Model file for the job. Use its own axes, mm. Coordinates: 2 decimals unless noted, no trailing zeros. Write each loop counter-clockwise with the first axis right and the second up, starting at its lowest first coordinate (ties: lowest second). Pieces come first, ordered by that corner, then holes.
Q1. Band-saw the part on A-A, the plane x = 25.4. Write the cut outline in (y, z) (1 decimal).
Q2. Band-saw the part on C-C, the plane y = -1.1. State how many separate pieces and enclosed holes the cut face has, plus the area to 3 significant figures.
Q3. Drill centre lines: probe 1 along X at (y, z) = (-2.25, -12.7); probe 2 along Z at (x, y) = (43.5, -2.65); probe 3 along X at (y, z) = (-2.1, -88) (3 decimals). Where is each one in solid material? Low to high.
Q4. Band-saw the part on B-B, the plane z = -12.7. Write the cut outline in (x, y) (3 decimals).
Q5. Band-saw the part on D-D, the plane x = 38.1. Write the cut outline in (y, z) (1 decimal), plus the area to 3 significant figures.
Q6. Pin check, flat tips, straight feed: P1, Ø1.6, axis at y = -1.5, z = -61, coming from the -X side (3 decimals); P2, Ø1, axis at x = 8, y = -1, coming from the -Z side; P3, Ø8, axis at x = 50.8, z = -87.31, coming from the +Y side; P4, Ø1.6, axis at y = -2, z = -85, coming from the -X side (3 decimals). Stop position of each tip, or through.
from build123d import *

# Parameters (mm, degrees)
SKETCH1_W          = 82.55
SKETCH1_H          = 96.8375
SKETCH1_W_2        = 38.1
SKETCH1_H_2        = 38.1
BASE_FLANGE2_DEPTH = 3.175
SKETCH3_W          = 12.7
SKETCH3_H          = 71.4375
CUT_EXTRUDE2_DEPTH = 128.287409162
SKETCH2_R          = 2.54
CUT_EXTRUDE1_DEPTH = 128.287409162
SKETCH5_W          = 15.875
SKETCH5_H          = 53.975
CUT_EXTRUDE6_DEPTH = 128.287409162
SKETCH7_R          = 2.54
CUT_EXTRUDE7_DEPTH = 128.287409162


# Sheet-metal steps are written as plain solids
with BuildPart() as part:
    # Base-Flange2: sheet metal written as solids
    # Sketch1 → Base-Flange2 (new body)
    with BuildSketch(Plane(origin=(0, 0, 0), x_dir=(1, 0, 0), z_dir=(0, 1, 0))):
        with Locations((41.275, 48.41875)):
            Rectangle(SKETCH1_W, SKETCH1_H)
        with Locations((47.625, 61.9125)):
            Rectangle(SKETCH1_W_2, SKETCH1_H_2, mode=Mode.SUBTRACT)
    extrude(amount=-BASE_FLANGE2_DEPTH)

    # Sketch3 → Cut-Extrude2 (cut, through all)
    with BuildSketch(Plane(origin=(0, 0, 0), x_dir=(1, 0, 0), z_dir=(0, 1, 0))):
        with Locations((6.35, 61.11875)):
            Rectangle(SKETCH3_W, SKETCH3_H)
    extrude(amount=-CUT_EXTRUDE2_DEPTH, mode=Mode.SUBTRACT)

    # Sketch2 → Cut-Extrude1 (cut, through all)
    with BuildSketch(Plane(origin=(0, 0, 0), x_dir=(1, 0, 0), z_dir=(0, 1, 0))):
        with Locations(Location((12.7, 12.7, 0), (0, 0, 270))):
            Circle(SKETCH2_R)
        with Locations(Location((25.4, 12.7, 0), (0, 0, 270))):
            Circle(SKETCH2_R)
        with Locations(Location((38.1, 12.7, 0), (0, 0, 270))):
            Circle(SKETCH2_R)
        with Locations(Location((50.8, 12.7, 0), (0, 0, 270))):
            Circle(SKETCH2_R)
    extrude(amount=-CUT_EXTRUDE1_DEPTH, mode=Mode.SUBTRACT)

    # Sketch5 → Cut-Extrude6 (cut, through all)
    with BuildSketch(Plane(origin=(0, 0, 0), x_dir=(1, 0, 0), z_dir=(0, 1, 0))):
        with Locations((20.6375, 69.85)):
            Rectangle(SKETCH5_W, SKETCH5_H)
    extrude(amount=-CUT_EXTRUDE6_DEPTH, mode=Mode.SUBTRACT)

    # Sketch7 → Cut-Extrude7 (cut, through all)
    with BuildSketch(Plane(origin=(0, 0, 0), x_dir=(1, 0, 0), z_dir=(0, 1, 0))):
        with Locations(Location((38.1, 87.3125, 0), (0, 0, 270))):
            Circle(SKETCH7_R)
        with Locations(Location((50.8, 87.3125, 0), (0, 0, 270))):
            Circle(SKETCH7_R)
    extrude(amount=-CUT_EXTRUDE7_DEPTH, mode=Mode.SUBTRACT)


solid = part.part
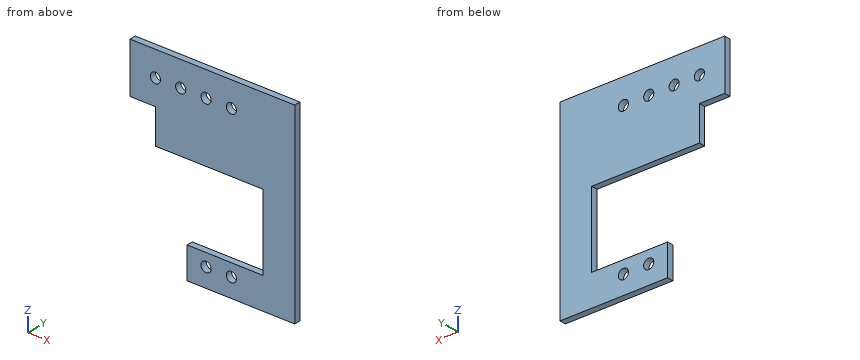
Answer sheet:
1. outline: (-3.2, -42.9) - (0, -42.9) - (0, -15.2) - (-3.2, -15.2) - close; (-3.2, -10.2) - (0, -10.2) - (0, 0) - (-3.2, 0) - close
2. separate pieces: 1
2. enclosed holes: 6
2. area: 4,660 mm2
3. probe 1: x = 0 to 10.16, 15.24 to 22.86, 27.94 to 35.56, 40.64 to 48.26, 53.34 to 82.55
3. probe 2: z = -96.84 to -80.96, -42.86 to 0
3. probe 3: x = 28.575 to 35.655, 40.545 to 48.355, 53.245 to 82.55
4. outline: (0, -3.175) - (10.16, -3.175) - (10.16, 0) - (0, 0) - close; (15.24, -3.175) - (22.86, -3.175) - (22.86, 0) - (15.24, 0) - close; (27.94, -3.175) - (35.56, -3.175) - (35.56, 0) - (27.94, 0) - close; (40.64, -3.175) - (48.26, -3.175) - (48.26, 0) - (40.64, 0) - close; (53.34, -3.175) - (82.55, -3.175) - (82.55, 0) - (53.34, 0) - close
5. outline: (-3.2, -96.8) - (0, -96.8) - (0, -89.9) - (-3.2, -89.9) - close; (-3.2, -84.8) - (0, -84.8) - (0, -81) - (-3.2, -81) - close; (-3.2, -42.9) - (0, -42.9) - (0, -15.2) - (-3.2, -15.2) - close; (-3.2, -10.2) - (0, -10.2) - (0, 0) - (-3.2, 0) - close
5. area: 154 mm2
6. P1: stops at x = 66.675
6. P2: stops at z = -25.4
6. P3: stops at y = 0
6. P4: stops at x = 28.575
